Could you check a few things on this model? Use its own coordinates, in mm. Face numbers are marked on the shaded views. A direction names the side the tool comes from. Give positions to 0.01 mm unless a question says otherwise; leave off trailing zeros. Order: outer loops, then holes, each group sorted by start corner. A loop starts at its lowest first (then second) coordinate and runs counter-clockwise, first axis right, second up. Notation, with made-up numbers: (-39, 59.25) -> (4, 59.25) arc R18 cw to (4, 66.25) -> close; hole circle Ø11 at (6, -23.75). An arc over 180 degrees is marked (long way). Answer as CSV lines item,"result". Start each with the question number.
(1) On a 3-axis mill with a long thin cutter (end or side, diameter ignored), from which of +Z, -Z, +X, -X, +Y, -Y can I reach the whole of each face in a straight line? I mean the marked faces 1 and 2. Say none if no direction works.
(2) I want a section at C-C (z = 0). Please give me the cut outline in (x, y), plus the area to 3 significant figures.
(3) Will these pins go through, and if not, where does the flat tip stop? pin 1 Ø1.5 at (y, z) = (2, 0.5) entering from -X; pin 2 Ø2.5 at (x, y) = (0, 0) entering from -Z; pin 3 Ø1.5 at (y, z) = (-1, -1) entering from +X.
(4) I need wall thicknesses on L1, parallel to X at y = 0, z = 0.5; L2, parallel to X at y = 1, z = -1.2. Which ranges of each line are inside material? Lowest first, please.
(5) We'd pull the mould along X, two halves only. Please class the marked faces 3, 4, 5 and 6: released by +X, released by -X, zero draft, split by the parting line, or undercut.
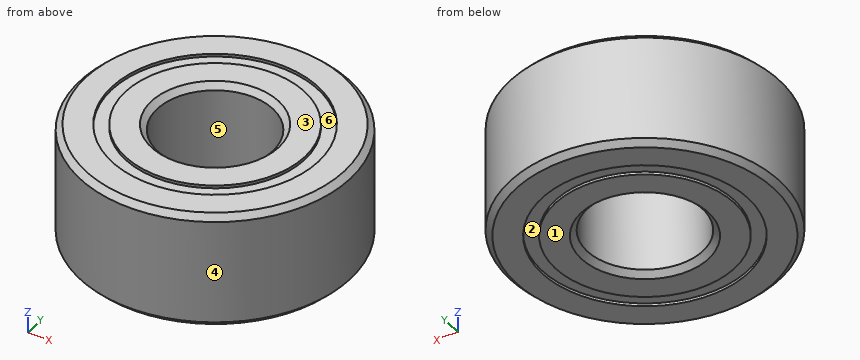
```python
from build123d import *

# Parameters (mm, degrees)
CHAMFER1_SIZE = 0.15


with BuildPart() as part:
    # Sketch3 → Revolve1 (revolve)
    with BuildSketch(Plane(origin=(0, 0, 0), x_dir=(1, 0, 0), z_dir=(0, 1, 0))):
        Polygon((1.5, -1.5), (1.5, 1.5), (2.325, 1.5), (2.325, 1.425), (2.675, 1.425), (2.675, 1.5), (3.5, 1.5), (3.5, -1.5), (2.675, -1.5), (2.675, -1.425), (2.325, -1.425), (2.325, -1.5), align=None)
    revolve(axis=Axis((0, 0, 0), (0, 0, -1)))

    # Chamfer1
    chamfer1_edges = [part.edges().sort_by_distance(p)[0] for p in [
        (-3.5, 0, 1.5),
        (-3.5, 0, -1.5),
        (-1.5, 0, -1.5),
        (-1.5, 0, 1.5),
    ]]
    chamfer(chamfer1_edges, length=CHAMFER1_SIZE)


solid = part.part
```
Final values:
1,face 1,"-Z, +X, -X, +Y, -Y"
1,face 2,"-Z"
2,outline,"circle Ø7 at (0, 0); hole circle Ø3 at (0, 0)"
2,area,"31.4 mm²"
3,pin 1,"x = -3.27"
3,pin 2,"through"
3,pin 3,"x = 3.49"
4,L1,"-3.5 to -1.5, 1.5 to 3.5"
4,L2,"-3.35 to -1.12, 1.12 to 3.35"
5,face 3,"zero draft"
5,face 4,"split by the parting line"
5,face 5,"undercut"
5,face 6,"undercut"
